Geometry: final body of the model. Coordinates: model frame, mm. A direction names the side the tool comes from. Give positions to 0.01 mm unless a question says otherwise; leave off trailing zeros. Write each loop counter-clockwise with the first axis right and the second up, starting at its lowest first coordinate (ties: lowest second). Pieces come first, ordered by that corner, then holes.
Q1. Pin query (flat end, axial travel): pin 1 (0.5 mm diameter, centred on x = 50.5, y = -3.5, fed in from -Z); pin 2 (10 mm diameter, centred on x = 33, y = 26, fed in from +Z). Return the tip coordinate at first contact, or that it passes through.
Q2. Line query: L1, parallel to Y at x = -29, z = 1.55; L2, parallel to Y at x = -42, z = 20.75; L3, parallel to X at y = 30, z = 11.5. Output: solid intervals per line, ascending.
Q3. Cut plane D-D on y = -21. Return the cut outline in (x, z), plus the area to 3 significant figures.
Q4. Cut plane B-B on x = 29. Return the cut outline in (y, z), plus the area to 3 significant figures.
Q5. Cut plane C-C on z = 8. Return the cut outline in (x, y).
Q6. Reachability of faces 1 (the face through (-1, 31.5, 12)), 2 (the face through (-49, 19, 17.6)), 3 (the face through (50, 0, 10)), 4 (the face through (51, 0, 22)) from +Z, -Z, +X, -X, +Y, -Y: full face, straight path, thin tool, end or side. Return the list, or none.
Q7. Draft query along Z for faces 5 (the face through (-29.303, -25.617, 1.521)), 6 (the face through (-49, -18, 17.3)), 7 (the face through (-49, -6.5, 10)). Return one class per face: pulls with the +Z half, pulls with the -Z half, needs draft (parallel to the pull), parting line crosses it, or undercut.
Q8. Cut plane A-A on y = 24.25. Return the cut outline in (x, z), plus the area to 3 significant figures.
```python
from build123d import *

# Parameters (mm, degrees)
SKETCH2_W           = 100
SKETCH2_H           = 67
BOSS_EXTRUDE1_DEPTH = 3
SKETCH3_W           = 100
SKETCH3_H           = 67
BOSS_EXTRUDE2_DEPTH = 21
SKETCH4_W           = 96
SKETCH4_H           = 63
CUT_EXTRUDE1_DEPTH  = 21
SKETCH5_R           = 1.4
CUT_EXTRUDE2_DEPTH  = 3
SKETCH9_W           = 14.3
SKETCH9_H           = 13
SKETCH9_H_2         = 12.7
SKETCH9_W_2         = 14.6
SKETCH9_H_3         = 15.3
CUT_EXTRUDE5_DEPTH  = 2
CUT_EXTRUDE7_START  = -100
SKETCH12_W          = 2
SKETCH12_H          = 65.6
CUT_EXTRUDE7_DEPTH  = 100
SKETCH16_W          = 3.920339225
SKETCH16_H          = 67
BOSS_EXTRUDE3_DEPTH = 1


with BuildPart() as part:
    # Sketch2 → Boss-Extrude1 (new body)
    with BuildSketch(Plane.XY):
        Rectangle(SKETCH2_W, SKETCH2_H)
    extrude(amount=BOSS_EXTRUDE1_DEPTH)

    # Sketch3 → Boss-Extrude2 (add)
    with BuildSketch(Plane.XY.offset(3)):
        Rectangle(SKETCH3_W, SKETCH3_H)
    extrude(amount=BOSS_EXTRUDE2_DEPTH)

    # Sketch4 → Cut-Extrude1 (cut)
    with BuildSketch(Plane.XY.offset(24)):
        Rectangle(SKETCH4_W, SKETCH4_H)
    extrude(amount=-CUT_EXTRUDE1_DEPTH, mode=Mode.SUBTRACT)

    # Sketch5 → Cut-Extrude2 (cut)
    with BuildSketch(Plane.XY.offset(3)):
        with Locations((-29, 24.25)):
            Circle(SKETCH5_R)
        with Locations((29, 24.25)):
            Circle(SKETCH5_R)
        with Locations((29, -24.25)):
            Circle(SKETCH5_R)
        with Locations((-29, -24.25)):
            Circle(SKETCH5_R)
    extrude(amount=-CUT_EXTRUDE2_DEPTH, mode=Mode.SUBTRACT)

    # Sketch9 → Cut-Extrude5 (cut)
    with BuildSketch(Plane.ZY.offset(50)):
        with Locations((10.15, -18.1)):
            Rectangle(SKETCH9_W, SKETCH9_H)
        with Locations((10.15, -0.15)):
            Rectangle(SKETCH9_W, SKETCH9_H_2)
        with Locations((10.3, 19.05)):
            Rectangle(SKETCH9_W_2, SKETCH9_H_3)
    extrude(amount=-CUT_EXTRUDE5_DEPTH, mode=Mode.SUBTRACT)

    # Sketch12 → Cut-Extrude7 (cut)
    with BuildSketch(Plane(origin=(50, 0, 0), x_dir=(0, 0, -1), z_dir=(1, 0, 0)).offset(CUT_EXTRUDE7_START)):
        with Locations((-22, 0)):
            Rectangle(SKETCH12_W, SKETCH12_H)
    extrude(amount=CUT_EXTRUDE7_DEPTH, mode=Mode.SUBTRACT)

    # Sketch16 → Boss-Extrude3 (add)
    with BuildSketch(Plane(origin=(50, 0, 0), x_dir=(0, 0, -1), z_dir=(1, 0, 0))):
        with Locations((-22.039830388, 0)):
            Rectangle(SKETCH16_W, SKETCH16_H)
    extrude(amount=BOSS_EXTRUDE3_DEPTH)


solid = part.part
```
Data:
1. pin 1: stops at z = 20.08
1. pin 2: stops at z = 3
2. L1: y = -33.5 to -25.65, -22.85 to 22.85, 25.65 to 33.5
2. L2: y = -33.5 to -31.5, 31.5 to 33.5
2. L3: x = -50 to -48, 48 to 50
3. outline: (-50, 0) - (50, 0) - (50, 20.08) - (51, 20.08) - (51, 24) - (48, 24) - (48, 23) - (50, 23) - (50, 21) - (48, 21) - (48, 3) - (-50, 3) - close; (-50, 17.3) - (-48, 17.3) - (-48, 21) - (-50, 21) - close; (-50, 23) - (-48, 23) - (-48, 24) - (-50, 24) - close
3. area: 351 mm2
4. outline: (-33.5, 0) - (-25.65, 0) - (-25.65, 3) - (-31.5, 3) - (-31.5, 21) - (-32.8, 21) - (-32.8, 23) - (-31.5, 23) - (-31.5, 24) - (-33.5, 24) - close; (-22.85, 0) - (22.85, 0) - (22.85, 3) - (-22.85, 3) - close; (25.65, 0) - (33.5, 0) - (33.5, 24) - (31.5, 24) - (31.5, 23) - (32.8, 23) - (32.8, 21) - (31.5, 21) - (31.5, 3) - (25.65, 3) - close
4. area: 263 mm2
5. outline: (-50, -33.5) - (50, -33.5) - (50, 33.5) - (-50, 33.5) - (-50, 26.7) - (-48, 26.7) - (-48, 31.5) - (48, 31.5) - (48, -31.5) - (-48, -31.5) - (-48, -24.6) - (-50, -24.6) - close; (-50, -11.6) - (-48, -11.6) - (-48, -6.5) - (-50, -6.5) - close; (-50, 6.2) - (-48, 6.2) - (-48, 11.4) - (-50, 11.4) - close
6. face 1: +Z
6. face 2: -X
6. face 3: -Z, +X, +Y, -Y
6. face 4: +Z, -Z, +X, +Y, -Y
7. face 5: needs draft
7. face 6: undercut
7. face 7: undercut
8. outline: (-50, 0) - (-30.4, 0) - (-30.4, 3) - (-50, 3) - close; (-50, 17.6) - (-48, 17.6) - (-48, 21) - (-50, 21) - close; (-50, 23) - (-48, 23) - (-48, 24) - (-50, 24) - close; (-27.6, 0) - (27.6, 0) - (27.6, 3) - (-27.6, 3) - close; (30.4, 0) - (50, 0) - (50, 20.08) - (51, 20.08) - (51, 24) - (48, 24) - (48, 23) - (50, 23) - (50, 21) - (48, 21) - (48, 3) - (30.4, 3) - close
8. area: 334 mm2
